```python
from build123d import *
from OCP.BRepFilletAPI import BRepFilletAPI_MakeChamfer

# Parameters (mm, degrees)
SKETCH_1_W               = 10.068208361
SKETCH_1_H               = 51.310344827
SKETCH_1_R               = 2
EXTRUDE_1_DEPTH          = 2.5
EXTRUDE_2_DEPTH          = 10.068208362
CUT_EXTRUDE_1_DEPTH      = 83.243670079
CUT_EXTRUDE_1_DEPTH_BACK = 83.243670079
CUT_EXTRUDE_2_DEPTH      = 122.121367623
CUT_EXTRUDE_2_DEPTH_BACK = 122.121367623
FILLET_2_R               = 2
CHAMFER_2_SIZE           = 2
CHAMFER_2_SIZE2          = 2.70532723


with BuildPart() as part:
    # 草图1 → 凸台-拉伸1 (new body)
    with BuildSketch(Plane.XY):
        with Locations((84.451834639, -55.007101597)):
            Rectangle(SKETCH_1_W, SKETCH_1_H)
        with Locations((84.623869854, -34.007101596)):
            Circle(SKETCH_1_R, mode=Mode.SUBTRACT)
        with Locations((84.623869854, -76.007101596)):
            Circle(SKETCH_1_R, mode=Mode.SUBTRACT)
    extrude(amount=EXTRUDE_1_DEPTH)

    # 草图2 → 凸台-拉伸2 (add)
    with BuildSketch(Plane(origin=(89.485938819, 0, 0), x_dir=(0, 0, -1), z_dir=(1, 0, 0))):
        Polygon((-12.5, -71.517171054), (-2.5, -73.914822505), (-2.5, -36.099380688), (-12.5, -38.497032139), align=None)
    extrude(amount=-EXTRUDE_2_DEPTH)

    # 草图3 → 切除-拉伸1 (cut, two sides: drawn at the far end of the back side and taken through both)
    with BuildSketch(Plane(origin=(89.485938819, 0, 0), x_dir=(0, 0, -1), z_dir=(1, 0, 0)).offset(-CUT_EXTRUDE_1_DEPTH_BACK)):
        Polygon((-10.198786391, -69.151033694), (0, -71.395312685), (0, -38.618890508), (-10.198786391, -40.863169498), align=None)
    extrude(amount=CUT_EXTRUDE_1_DEPTH + CUT_EXTRUDE_1_DEPTH_BACK, mode=Mode.SUBTRACT)

    # 草图4 → 切除-拉伸2 (cut, two sides: drawn at the far end of the back side and taken through both)
    with BuildSketch(Plane.XY.offset(12.5).offset(-CUT_EXTRUDE_2_DEPTH_BACK)):
        with BuildLine():
            Line((81.544440974, -36.941486908), (81.544440974, -73.072716285))
            ThreePointArc((81.544440974, -73.072716285), (79.417730458, -75.199426802), (77.291019941, -73.072716285))
            Line((77.291019941, -73.072716285), (77.291019941, -36.941486908))
            ThreePointArc((77.291019941, -36.941486908), (79.417730458, -34.814776391), (81.544440974, -36.941486908))
        make_face()
        with BuildLine():
            Line((87.359228302, -36.941486908), (87.359228302, -73.072716285))
            ThreePointArc((87.359228302, -73.072716285), (89.485938819, -75.199426802), (91.612649336, -73.072716285))
            Line((91.612649336, -73.072716285), (91.612649336, -36.941486908))
            ThreePointArc((91.612649336, -36.941486908), (89.485938819, -34.814776391), (87.359228302, -36.941486908))
        make_face()
    extrude(amount=CUT_EXTRUDE_2_DEPTH + CUT_EXTRUDE_2_DEPTH_BACK, mode=Mode.SUBTRACT)

    # 圆角1
    # a fillet whose section is not a circle: 3 mm, written as the material it adds along each edge
    with BuildSketch(Plane(origin=(87.359228302, -40.863169498, 10.198786391), x_dir=(0, 0.2149116520268582, -0.9766334941128564), z_dir=(-1, 0, 0)), Plane(origin=(87.359228302, -69.151033694, 10.198786391), x_dir=(0, 1, 0), z_dir=(-1, 0, 0))) as fillet_1_piece_1:
        with BuildLine():
            Bezier((2.411616085, 0), (0, 0), (-0.518284397, 2.355265044), weights=[1, 0.666666667, 1])
            Line((-0.518284397, 2.355265044), (0, 0))
            Line((0, 0), (2.411616085, 0))
        make_face()
    extrude(amount=5.814787328)

    # 圆角2
    fillet_2_edges = [part.edges().sort_by_distance(p)[0] for p in [
        (89.485938819, -80.66227401, 1.25),
        (79.417730458, -80.66227401, 1.25),
        (79.417730458, -29.351929183, 1.25),
        (89.485938819, -29.351929183, 1.25),
    ]]
    fillet(fillet_2_edges, radius=FILLET_2_R)

    # 倒角2: one chamfer whose edges measure the first distance from different faces: ONE call of the kernel's chamfer builder (chamfer() names one face for all edges)
    chamfer_2_edges_1 = [part.edges().sort_by_distance(p)[0] for p in [
        (84.451834638, -71.517171054, 12.5),
    ]]
    chamfer_2_side_1 = [part.faces().sort_by_distance(p)[0] for p in [
        (84.451834638, -72.722762821, 7.471780545),
    ]]
    chamfer_2_edges_2 = [part.edges().sort_by_distance(p)[0] for p in [
        (84.451834638, -38.497032139, 12.5),
    ]]
    chamfer_2_side_2 = [part.faces().sort_by_distance(p)[0] for p in [
        (84.451834638, -55.007101596, 12.5),
    ]]
    chamfer_2 = BRepFilletAPI_MakeChamfer(part.part.solid().wrapped)
    for e in chamfer_2_edges_1:
        chamfer_2.Add(CHAMFER_2_SIZE, CHAMFER_2_SIZE2, e.wrapped, chamfer_2_side_1[0].wrapped)  # the first distance lies on this face
    for e in chamfer_2_edges_2:
        chamfer_2.Add(CHAMFER_2_SIZE, CHAMFER_2_SIZE2, e.wrapped, chamfer_2_side_2[0].wrapped)  # the first distance lies on this face
    add(Compound.cast(chamfer_2.Shape()), mode=Mode.REPLACE)


solid = part.part
```
Geometry: final body of the model. Coordinates: model frame, mm. A direction names the side the tool comes from. Give positions to 0.01 mm unless a question says otherwise; leave off trailing zeros. Loops run counter-clockwise (first coordinate to the right, second up) from the corner with the lowest first, then second, coordinate; pieces in that order, holes last. Notation, with made-up numbers: (24.5, 39.5) -> (68.5, 39.5) arc R17 cw to (68.5, 65.5) -> close; hole circle Ø4 at (26.25, 35). An arc over 180 degrees is marked (long way). Use CSV: the item, a comma, the result in double quotes.
(1) Pull-direction query (X, two-part tool) for faces 1 (the face through (86.532, -33.406, 1.232)), 2 (the face through (88.916, -80.061, 1.268)), 3 (the face through (80.905, -35.421, 1.628)); classes: released by +X, released by -X, zero draft, split by the parting line, or undercut.
From the geometry:
face 1,"undercut"
face 2,"released by +X"
face 3,"released by -X"
(2) Cut plane A-A (z = 1.5). Output: boundary loops of the cut face in (x, y).
From the geometry:
outline,"(79.42, -78.66) arc R2 ccw to (81.42, -80.66) -> (87.49, -80.66) arc R2 ccw to (89.49, -78.66) -> (89.49, -75.2) arc R2.13 cw to (87.36, -73.07) -> (87.36, -71.07) -> (81.54, -71.07) -> (81.54, -73.07) arc R2.13 cw to (79.42, -75.2) -> close; (79.42, -34.81) arc R2.13 cw to (81.54, -36.94) -> (81.54, -38.95) -> (87.36, -38.95) -> (87.36, -36.94) arc R2.13 cw to (89.49, -34.81) -> (89.49, -31.35) arc R2 ccw to (87.49, -29.35) -> (81.42, -29.35) arc R2 ccw to (79.42, -31.35) -> close; hole circle Ø4 at (84.62, -76.01); hole circle Ø4 at (84.62, -34.01)"
(3) Cut plane D-D (x = 83.5). Count the separate pieces of the cut face and the enclosed holes in it, plus the area to 3 significant figures.
From the geometry:
separate pieces,"3"
enclosed holes,"0"
area,"152 mm^2"
(4) Access query for faces 4 (the face through (84, -79, 2.5)), 5 (the face through (81.544, -55, 11)), 6 (the face through (84.41, -39.47, 3.87)). Directions: +Z, -Z, +X, -X, +Y, -Y. A direction counts if a zero-diameter tool reaches every point of the face in a straight line with its end or side. Return the directions, or none.
From the geometry:
face 4,"+Z, +X, -X, -Y"
face 5,"+Z, -Z, -X"
face 6,"-Z, +X, -X"
(5) Ray query, line 1 along Y through (x, z) = (85.5, 1.75); line 2 along Y through (x, z) = (86, 9.25); line 3 along X through (y, z) = (-48, 10.25). Return the intervals inside material, ascending. Write a range as [from, to].
From the geometry:
line 1,"[-80.66, -77.8], [-74.21, -71.01], [-39, -35.8], [-32.21, -29.35]"
line 2,"[-72.3, -68.85], [-41.16, -37.72]"
line 3,"[81.54, 87.36]"
(6) Cut plane B-B (x = 88.25). Output: boundary loops of the cut face in (y, z), plus the area to 3 significant figures.
From the geometry:
outline,"(-80.51, 0) -> (-74.8, 0) -> (-74.8, 2.5) -> (-80.51, 2.5) -> close; (-35.21, 0) -> (-29.5, 0) -> (-29.5, 2.5) -> (-35.21, 2.5) -> close"
area,"28.5 mm^2"
(7) First-contact query: P1, Ø4.5, axis at x = 84.5, y = -49.5, coming from the -Z side; P2, Ø5, axis at x = 84.62, y = -76.01, coming from the -Z side; P3, Ø3.5, axis at x = 86, y = -34, coming from the +Z side; P4, Ø6, axis at x = 85, y = -73.5, coming from the +Z side. Flat tips, straight axial feed; report the tip coordinate or a pass-through.
From the geometry:
P1,"z = 10.2"
P2,"z = 0"
P3,"z = 2.5"
P4,"z = 11.46"
(8) Cut plane C-C (z = 5.5). Output: boundary loops of the cut face in (x, y), plus the area to 3 significant figures.
From the geometry:
outline,"(81.54, -73.2) -> (87.36, -73.2) arc R2.13 cw to (87.36, -73.07) -> (87.36, -70.19) -> (81.54, -70.19) -> (81.54, -73.07) arc R2.13 cw to start; (81.54, -39.83) -> (87.36, -39.83) -> (87.36, -36.94) arc R2.13 cw to (87.36, -36.82) -> (81.54, -36.82) arc R2.13 cw to (81.54, -36.94) -> close"
area,"35.0 mm^2"
